from build123d import *

# Parameters (mm, degrees)
F0_R     = 4.7625
F1_DEPTH = 6.35
F2_SIZE  = 1.1
F3_DEPTH = 6.35
F4_DEPTH = 45
F5_SIZE  = 1


# Not quite as in the source:
# - a length typed as a fraction of an inch, garbled in the dataset ("3 / 203.2 mm" for 3/8 in), is restored


with BuildPart() as f1:
    # F0 (on Top) → F1 (new body)
    with BuildSketch(Plane.XY):
        with BuildLine():
            ThreePointArc((0, -8.248891971), (4.1244459855, -7.14375), (7.14375, -4.1244459855))
            Line((7.14375, -4.1244459855), (0, -8.248891971))
        make_face()
        with BuildLine():
            ThreePointArc((8.248891971, 0), (7.9678177931, 2.1349703431), (7.14375, 4.1244459855))
            Line((7.14375, 4.1244459855), (7.14375, -4.1244459855))
            ThreePointArc((7.14375, -4.1244459855), (7.9678177931, -2.1349703431), (8.248891971, 0))
        make_face()
        with BuildLine():
            Line((0, 8.248891971), (7.14375, 4.1244459855))
            ThreePointArc((7.14375, 4.1244459855), (4.1244459855, 7.14375), (0, 8.248891971))
        make_face()
        with BuildLine():
            Line((-7.14375, 4.1244459855), (0, 8.248891971))
            ThreePointArc((0, 8.248891971), (-4.1244459855, 7.14375), (-7.14375, 4.1244459855))
        make_face()
        Polygon((7.14375, -4.1244459855), (7.14375, 4.1244459855), (0, 8.248891971), (-7.14375, 4.1244459855), (-7.14375, -4.1244459855), (0, -8.248891971), align=None)
        Circle(F0_R, mode=Mode.SUBTRACT)
        Circle(F0_R)
        with BuildLine():
            Line((-7.14375, -4.1244459855), (-7.14375, 4.1244459855))
            ThreePointArc((-7.14375, 4.1244459855), (-8.248891971, 0), (-7.14375, -4.1244459855))
        make_face()
        with BuildLine():
            ThreePointArc((-7.14375, -4.1244459855), (-4.1244459855, -7.14375), (0, -8.248891971))
            Line((0, -8.248891971), (-7.14375, -4.1244459855))
        make_face()
    extrude(amount=F1_DEPTH)

    # F2
    f2_edges = [f1.edges().sort_by_distance(p)[0] for p in [
        (7.14375, 4.124446, 6.35),
    ]]
    chamfer(f2_edges, length=F2_SIZE)

    # F0 (on Top) → F3 (intersect)
    with BuildSketch(Plane.XY):
        Polygon((7.14375, -4.1244459855), (7.14375, 4.1244459855), (0, 8.248891971), (-7.14375, 4.1244459855), (-7.14375, -4.1244459855), (0, -8.248891971), align=None)
        Circle(F0_R, mode=Mode.SUBTRACT)
        Circle(F0_R)
    extrude(amount=F3_DEPTH, mode=Mode.INTERSECT)

    # F0 (on Top) → F4 (join)
    with BuildSketch(Plane.XY):
        Circle(F0_R)
    extrude(amount=-F4_DEPTH)

    # F5
    f5_edges = [f1.edges().sort_by_distance(p)[0] for p in [
        (-4.7625, 0, -45),
    ]]
    chamfer(f5_edges, length=F5_SIZE)


solid = f1.part
Work out the finished part from the listing and answer in its coordinate system (mm). A direction names the side the tool comes from. Round coordinates to 2 decimals unless told otherwise and drop trailing zeros. Order: outer loops, then holes, each group sorted by start corner. A loop starts at its lowest first (then second) coordinate and runs counter-clockwise, first axis right, second up. Notation, with made-up numbers: M -25,80 L -17,80 A27 ccw -17,119 Z; hole C 13.25,66 d1. An arc over 180 degrees is marked long. One line per item, written item: value.
Q1. Flat-ended cylindrical pins translate along their axes: pin 1 (1.5 mm diameter, centred on x = 2.5, z = -21, fed in from -Y); pin 2 (4 mm diameter, centred on y = -0.5, z = -28.5, fed in from +X); pin 3 (1 mm diameter, centred on x = 1.5, z = -10.5, fed in from -Y). Find the tip coordinate at first contact, or state that the pin passes through.
Derived:
pin 1: y = -4.43
pin 2: x = 4.76
pin 3: y = -4.66
Q2. Find section A-A on z = -40.5. Write down the section's boundary in (x, y) (1 decimal).
Derived:
outline: C 0,0 d9.5
Q3. For faces 1 (the face through (-3, -4, 0)), 2 (the face through (3.522, -6.216, 3.131)), determine the directions among +Z, -Z, +X, -X, +Y, -Y from which every point of the face is accessible in a straight line to the end or side of a thin tool.
Derived:
face 1: -Z
face 2: +Z, -Z, +X, -Y
Q4. Straight lines are drawn through the part: line 1 (X direction, y = -0.25, z = -21); line 2 (Z direction, x = -2.5, y = -4.5); line 3 (Y direction, x = 2, z = -29). For each, find the intervals that lie inside material, in ascending order.
Derived:
line 1: -4.76 to 4.76
line 2: 0 to 6.35
line 3: -4.32 to 4.32
